Drawing for the job (mm, zero at the part's lowest x, y, z). A direction names the side the tool comes from. Give positions to 0.01 mm unless a question says otherwise; leave off trailing zeros. Loops run counter-clockwise (first coordinate to the right, second up) from the corner with the lowest first, then second, coordinate; pieces in that order, holes last. Notation, with made-up numbers: (-3.75, 85) -> (27.25, 85) arc R15 cw to (27.25, 106) -> close; hole circle Ø1 at (-2.5, 56). An arc over 180 degrees is marked (long way). Answer in a Markdown table with one row per item. Add a question column.
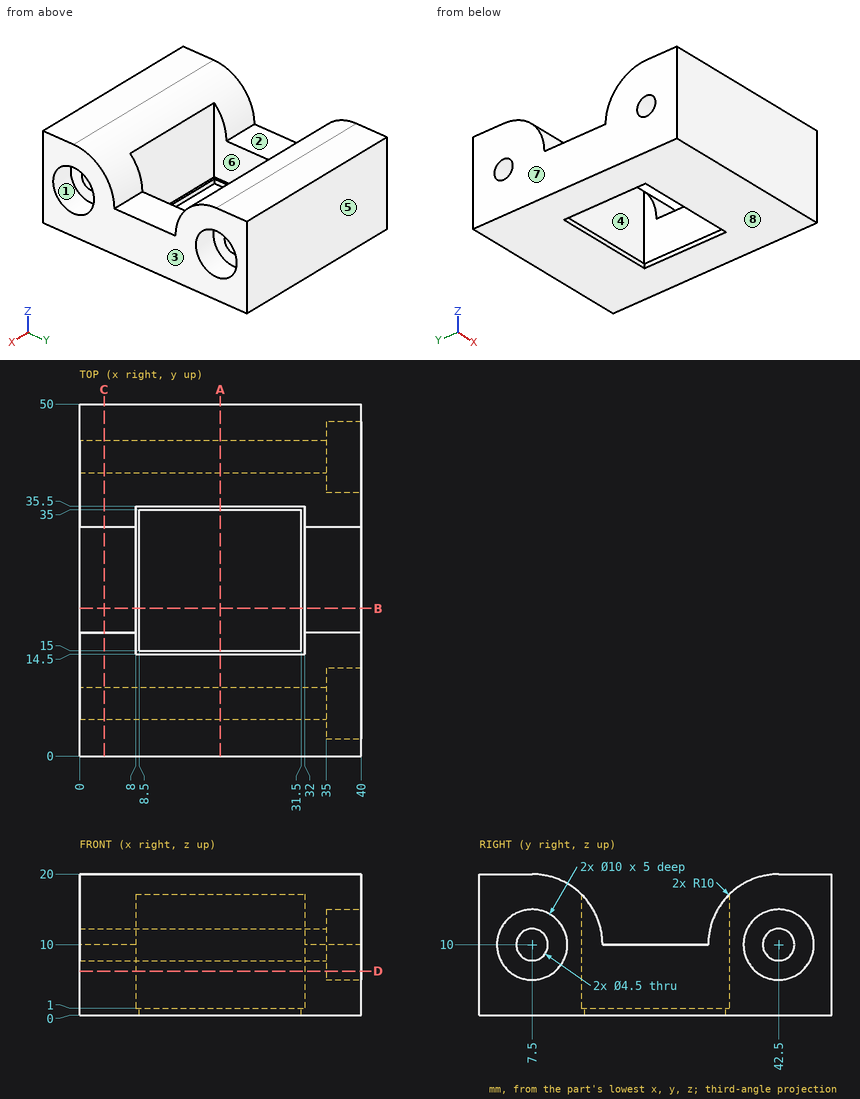
(1) Wall check: line 1 along Y through (x, z) = (29.5, 4); line 2 along Z through (x, y) = (21, 7.5); line 3 along X through (y, z) = (19.5, 1.75). Give the ranges that are in metal, low to high. Write a range as from..to.
(2) 3-axis set-ups, long thin cutter, end or side, ignore diameter. For the marked faces 1, 2, 3, 4 and 5: which of +Z, -Z, +X, -X, +Y, -Y reach the whole face in a straight line?
(3) Saw through at D-D, the plane z = 6.25. List the corners of the cut face in (x, y).
(4) Saw through at B-B, the plane y = 21. List the corners of the cut face in (x, z), then the cut area to 3 significant figures.
(5) Two-plate mould, pull along X, no slides. Class the marked faces 6, 7 and 8: released by +X, released by -X, zero draft, split by the parting line, or undercut.
(6) Flat gauge pins, fed straight in: pin 1 Ø3 at (y, z) = (9.5, 10) entering from +X; pin 2 Ø5 at (x, y) = (8.5, 24.5) entering from -Z; pin 3 Ø2.5 at (x, y) = (5.5, 22.5) entering from +Z. Where does each tip first touch, or does it go through?
(7) Saw through at A-A, the plane x = 20. List the corners of the cut face in (y, z).
(8) Saw through at C-C, the plane x = 3.5. List the corners of the cut face in (y, z), then the cut area to 3 significant figures.
Worked answers:
| question | item | result |
|---|---|---|
| 1 | line 1 | 0..14.5, 35.5..50 |
| 1 | line 2 | 0..7.75, 12.25..20 |
| 1 | line 3 | 0..8, 32..40 |
| 2 | face 1 | +X |
| 2 | face 2 | +Z, +X, -X |
| 2 | face 3 | +Z, -Z, +X, +Y, -Y |
| 2 | face 4 | +Z |
| 2 | face 5 | +Z, -Z, +X, -X, +Y |
| 3 | outline | (0, 0) -> (40, 0) -> (40, 4.19) -> (35, 4.19) -> (35, 10.81) -> (40, 10.81) -> (40, 39.19) -> (35, 39.19) -> (35, 45.81) -> (40, 45.81) -> (40, 50) -> (0, 50) -> close; hole (8, 14.5) -> (32, 14.5) -> (32, 35.5) -> (8, 35.5) -> close |
| 4 | outline | (0, 0) -> (8.5, 0) -> (8.5, 1) -> (8, 1) -> (8, 10) -> (0, 10) -> close; (31.5, 0) -> (40, 0) -> (40, 10) -> (32, 10) -> (32, 1) -> (31.5, 1) -> close |
| 4 | area | 161 mm^2 |
| 5 | face 6 | undercut |
| 5 | face 7 | released by -X |
| 5 | face 8 | zero draft |
| 6 | pin 1 | x = 35 |
| 6 | pin 2 | z = 0 |
| 6 | pin 3 | z = 10 |
| 7 | outline | (0, 0) -> (15, 0) -> (15, 1) -> (14.5, 1) -> (14.5, 17.14) arc R10 ccw to (7.5, 20) -> (0, 20) -> close; (35, 0) -> (50, 0) -> (50, 20) -> (42.5, 20) arc R10 ccw to (35.5, 17.14) -> (35.5, 1) -> (35, 1) -> close; hole circle Ø4.5 at (7.5, 10); hole circle Ø4.5 at (42.5, 10) |
| 8 | outline | (0, 0) -> (50, 0) -> (50, 20) -> (42.5, 20) arc R10 ccw to (32.5, 10) -> (17.5, 10) arc R10 ccw to (7.5, 20) -> (0, 20) -> close; hole circle Ø4.5 at (7.5, 10); hole circle Ø4.5 at (42.5, 10) |
| 8 | area | 775 mm^2 |
